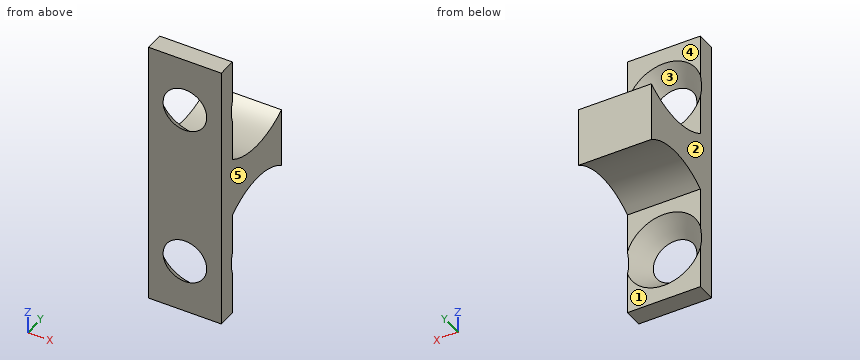
```python
from build123d import *

# Parameters (mm, degrees)
BOSS_EXTRUDE2_DEPTH                           = 6.746875
CUT_EXTRUDE1_REACH                            = 8.747
CSK_FOR_6_FLAT_HEAD_MACHINE_SCREW1_AT_2_COUNT = 2
CSK_FOR_6_FLAT_HEAD_MACHINE_SCREW1_AT_2_PITCH = 15.08125


with BuildPart() as part:
    # Sketch2 → Boss-Extrude2 (new body)
    with BuildSketch(Plane(origin=(0, 0, 0), x_dir=(0, 0, -1), z_dir=(1, 0, 0))):
        Polygon((-2.049136217, 1.594614568), (-11.782098717, 1.594614568), (-11.782098717, -0.132585432), (13.221026283, -0.132585432), (13.221026283, 1.620014568), (3.488063783, 1.620014568), (3.488063783, 9.265414568), (-2.049136217, 9.265414568), align=None)
    extrude(amount=BOSS_EXTRUDE2_DEPTH)

    # Sketch9 → Cut-Extrude1 (cut, up to next)
    with BuildSketch(Plane(origin=(6.746875, 0, 0), x_dir=(0, 0, -1), z_dir=(1, 0, 0)), mode=Mode.PRIVATE) as cut_extrude1_sk1:
        with BuildLine():
            Line((-2.049136217, 9.265414568), (-2.049136217, 1.594614568))
            ThreePointArc((-2.049136217, 1.594614568), (-0.958515707, 5.430014568), (-2.049136217, 9.265414568))
        make_face()
    cut_extrude1_tool1 = extrude(cut_extrude1_sk1.sketch, amount=-CUT_EXTRUDE1_REACH, mode=Mode.PRIVATE) & part.part
    add(cut_extrude1_tool1.solids().sort_by_distance((6.746875, 5.430015, 1.609964))[0], mode=Mode.SUBTRACT)
    # Sketch9 → Cut-Extrude1 (cut, up to next)
    with BuildSketch(Plane(origin=(6.746875, 0, 0), x_dir=(0, 0, -1), z_dir=(1, 0, 0)), mode=Mode.PRIVATE) as cut_extrude1_sk2:
        with BuildLine():
            Line((3.488063783, 9.265414568), (3.488063783, 1.620014568))
            ThreePointArc((3.488063783, 1.620014568), (2.281768381, 5.442714568), (3.488063783, 9.265414568))
        make_face()
    cut_extrude1_tool2 = extrude(cut_extrude1_sk2.sketch, amount=-CUT_EXTRUDE1_REACH, mode=Mode.PRIVATE) & part.part
    add(cut_extrude1_tool2.solids().sort_by_distance((6.746875, 5.442715, -3.001592))[0], mode=Mode.SUBTRACT)

    # Sketch7 → CSK for #6 Flat Head Machine Screw1 (revolve, cut)
    with BuildSketch(Plane(origin=(3.374760147, 1.620014568, -8.260088783), x_dir=(0, 0, 1), z_dir=(1, 0, 0))):
        Polygon((0, 0), (0, 1.7526), (1.89865, 1.7526), (1.89865, 1.891953401), (3.5433, 0), align=None)
    csk_for_6_flat_head_machine_screw1 = revolve(axis=Axis((3.374760147, 7.970014568, -8.260088783), (0, -1, 0)), mode=Mode.SUBTRACT)

    # CSK for #6 Flat Head Machine Screw1 at 2: CSK for #6 Flat Head Machine Screw1 ×2
    with Locations(*[Vector(-8.7701e-05, 0, 0.999999996) * (i * CSK_FOR_6_FLAT_HEAD_MACHINE_SCREW1_AT_2_PITCH) for i in range(1, CSK_FOR_6_FLAT_HEAD_MACHINE_SCREW1_AT_2_COUNT)]):
        add(csk_for_6_flat_head_machine_screw1, mode=Mode.SUBTRACT)


solid = part.part
```
For this review, take the finished solid that the model builds, in its own axes (mm). Face numbers are marked on the shaded views. A direction names the side the tool comes from. Round coordinates to 2 decimals unless told otherwise and drop trailing zeros. Loops run counter-clockwise (first coordinate to the right, second up) from the corner with the lowest first, then second, coordinate; pieces in that order, holes last.
(1) Tool access review of the marked faces 1 and 2: name each direction out of +Z, -Z, +X, -X, +Y, -Y from which nothing blocks a thin tool from reaching the whole face with its end or side.
Returned:
face 1: -Z, +X, -X, +Y
face 2: +Z, -Z, -X, +Y, -Y
(2) We need section B-B (x = 3.75). State how many separate pieces and enclosed holes the cut face has, plus the area to 3 significant figures.
Returned:
separate pieces: 3
enclosed holes: 0
area: 54.8 mm2
(3) Clearance check with flat-ended pins moving along their axes: P1, Ø3, axis at x = 4.5, y = 3, coming from the +Z side; P2, Ø3, axis at x = 3, z = 10, coming from the +Y side; P3, Ø1.8, axis at x = 3, z = -6, coming from the +Y side; P4, Ø4, axis at x = 2.5, y = 7.5, coming from the +Z side. State where each tip first meets the part, or that it passes through.
Returned:
P1: stops at z = 11.78
P2: stops at y = 1.59
P3: stops at y = 1.21
P4: stops at z = 2.05
(4) We need section C-C (z = -3.75). Give the boundary of the cut face in (x, y), plus the area to 3 significant figures.
Returned:
outline: (0, -0.13) - (6.75, -0.13) - (6.75, 1.62) - (0, 1.62) - close
area: 11.8 mm2
(5) We need section A-A (y = 0.75). Give the boundary of the cut face in (x, z), plus the area to 3 significant figures.
Returned:
outline: (0, -13.22) - (6.75, -13.22) - (6.75, 11.78) - (0, 11.78) - close; hole circle Ø5.57 at (3.37, -8.26); hole circle Ø5.57 at (3.37, 6.82)
area: 120 mm2
(6) Mouldability with a two-part tool opening along X and no side actions: class the marked faces 3, 4 and 5 as released by +X, released by -X, zero draft, split by the parting line, or undercut.
Returned:
face 3: undercut
face 4: zero draft
face 5: released by +X
(7) We need section D-D (y = 3.5). Give the boundary of the cut face in (x, z).
Returned:
outline: (0, -2.57) - (6.75, -2.57) - (6.75, 1.22) - (0, 1.22) - close
(8) Wall thickness on line 1 along Z through (x, y) = (6, 1.25); line 2 along Y through (x, z) = (0.5, 4); line 3 along Z through (x, y) = (2, 1.25): over which ranges is each line inside the solid? List them lowest first.
Returned:
line 1: z = -13.22 to -10.13, -6.39 to 4.96, 8.69 to 11.78
line 2: y = -0.13 to 1.59
line 3: z = -13.22 to -11.17, -5.35 to 3.91, 9.74 to 11.78
